Input: part model. Units: mm. Frame: model coordinates. Face numbers are marked on the shaded views. A direction names the side the tool comes from. Coordinates: 2 decimals unless noted, no trailing zeros. Loops run counter-clockwise (first coordinate to the right, second up) from the corner with the lowest first, then second, coordinate; pieces in that order, holes last. Notation, with made-up numbers: (38.25, 55.5) - (89.25, 55.5) arc R20 cw to (89.25, 72.5) - close; hole circle Ø2 at (-4.5, 1.25). An arc over 180 degrees is marked (long way). Use a Markdown table: item, result. Add a question column.
1. Draft query along X for the marked faces 3 and 4. Return one class per face: released by +X, released by -X, zero draft, split by the parting line, or undercut.
2. Section query B-B on y = 50.5. Return the cut outline in (x, z).
3. Section query C-C on y = 23. Return the cut outline in (x, z).
4. Ray query, L1, parallel to Y at x = -49, z = 1.4; L2, parallel to Y at x = -20, z = 0.55; L3, parallel to X at y = 54, z = 1.5. Return the intervals inside material, ascending. Write a range as [from, to].
5. Access query for the marked faces 1 and 2. Directions: +Z, -Z, +X, -X, +Y, -Y. A direction counts if a zero-diameter tool reaches every point of the face in a straight line with its end or side. Return the directions, or none.
6. Section query D-D on x = -4. Return the cut outline in (y, z).
7. Contact query for flat-ended pins moving along their axis: P1, Ø1, axis at x = -47.5, y = 53, coming from the +Z side; P2, Ø0.9, axis at x = -61, z = 2, coming from the -Y side; P3, Ø0.9, axis at x = -10.5, z = 1.5, coming from the -Y side; P4, Ø1.4, axis at x = -3.5, z = 1, coming from the -Y side. Output: stop coordinate, or through.
8. Section query A-A on x = -39.5. State how many separate pieces and enclosed holes the cut face has, then the cut area to 3 significant figures.
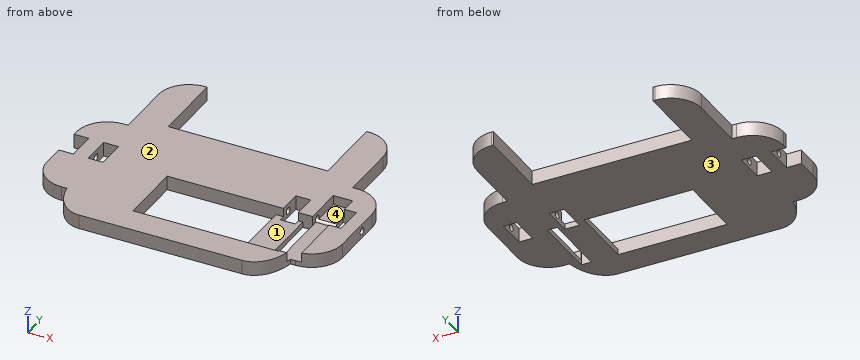
Autodesk Inventor part; units mm, degrees
ref_plane "YZ Plane" through (0, 0, 0) normal (1, 0, 0) x (0, 1, 0)
ref_plane "XZ Plane" through (0, 0, 0) normal (0, 1, 0) x (-1, 0, 0)
ref_plane "XY Plane" through (0, 0, 0) normal (0, 0, 1) x (1, 0, 0)
ref_plane "Work Plane1" through (3.6062, 5.0251, 0) normal (0, 0, 1) x (1, 0, 0)
sketch "Sketch1" plane through (3.6062, 5.0251, 0) normal (0, 0, 1) x (1, 0, 0)
  line L0 (-59.3453, 14.0249) -> (-60.5022, 14.0249)
  ellipse E0 centre (-52.8822, 15.9436) end of major axis (-52.8822, 6.6041) minor radius 6.604 (-59.3453, 14.0249) -> (-52.8822, 6.6041) ccw
  line L1 (-52.8822, 6.6041) -> (-17.8302, 6.6041)
  ellipse E1 centre (-17.8302, 15.9436) end of major axis (-17.8302, 25.2831) minor radius 6.604 (-17.8302, 6.6041) -> (-11.367, 14.0249) ccw
  line L2 (-10.2102, 14.0249) -> (-11.367, 14.0249)
  arc A0 (-10.2102, 14.0249) -> (-3.6062, 20.6289) centre (-10.2102, 20.6289) ccw
  line L3 (-3.6062, 20.6289) -> (-3.6062, 32.8209)
  arc A1 (-3.6062, 32.8209) -> (-10.2102, 39.4249) centre (-10.2102, 32.8209) ccw
  line L4 (-11.2262, 39.4249) -> (-10.2102, 39.4249)
  line L5 (-11.2262, 51.8709) -> (-11.2262, 39.4249)
  arc A2 (-11.2262, 51.8709) -> (-17.8302, 58.4749) centre (-17.8302, 51.8709) ccw
  line L6 (-17.8302, 58.4749) -> (-52.8822, 58.4749)
  arc A3 (-52.8822, 58.4749) -> (-59.4862, 51.8709) centre (-52.8822, 51.8709) ccw
  line L7 (-59.4862, 39.4249) -> (-59.4862, 51.8709)
  line L8 (-60.5022, 39.4249) -> (-59.4862, 39.4249)
  arc A4 (-60.5022, 39.4249) -> (-67.1062, 32.8209) centre (-60.5022, 32.8209) ccw
  line L9 (-67.1062, 20.6289) -> (-67.1062, 32.8209)
  arc A5 (-67.1062, 20.6289) -> (-60.5022, 14.0249) centre (-60.5022, 20.6289) ccw
  line L10 (-52.8822, 6.6041) -> (-17.8302, 6.6041)
  point P0 (-3.6062, -5.0251)
extrude "Plate1" add sketch "Sketch1" along normal blind 3.048
sketch "Sketch2" plane through (3.6062, 5.0251, 3.048) normal (0, 0, 1) x (1, 0, 0)
  line L0 (-19.2272, 69.2699) -> (-19.2272, 51.2359)
  line L1 (-42.2142, 43.5397) -> (-28.4982, 43.5397)
  line L2 (-51.4852, 51.2359) -> (-51.4852, 69.2699)
  line L3 (-19.2272, 58.5208) -> (-19.2272, 43.5397)
  line L4 (-19.2272, 43.5397) -> (-51.4852, 43.5397)
  line L5 (-51.4852, 43.5397) -> (-51.4852, 64.3147)
  line L6 (-52.4852, 58.4749) -> (-52.4852, 42.5397)
  line L7 (-52.4852, 42.5397) -> (-18.2272, 42.5397)
  line L8 (-18.2272, 42.5397) -> (-18.2272, 58.5208)
  line L9 (-52.8822, 58.4749) -> (-17.8302, 58.4749)
  point P0 (0, 0)
  point P1 (-18.2272, 58.4749)
  dimension "d2" = 1
extrude "Extrusion2" cut sketch "Sketch2" against normal through all
sketch "Sketch4" plane through (3.6062, 5.0251, 3.048) normal (0, 0, 1) x (1, 0, 0)
  line L0 (-12.8862, 21.4549) -> (-12.8862, 17.4549)
  line L1 (-9.0098, 35.2125) -> (-13.2052, 35.2125)
  line L2 (-13.2052, 35.2125) -> (-13.2052, 18.2304)
  line L3 (-13.2052, 18.2304) -> (-12.8862, 18.2304)
  line L4 (-9.0098, 16.8588) -> (-9.0098, 35.2125)
  line L5 (-9.0098, 35.2125) -> (-13.2052, 18.2304) construction
  line L6 (-13.2052, 35.2125) -> (-9.0098, 16.8588) construction
  line L7 (-12.8862, 21.4549) -> (-12.8862, 17.4549)
  line L8 (-3.6062, 30.2174) -> (-8.2582, 30.2174)
  line L9 (-12.8862, 17.9549) -> (-3.6562, 17.9549)
  line L10 (-12.8862, 21.4549) -> (-12.8862, 17.4549)
  line L11 (-13.2052, 18.2304) -> (-12.8862, 18.2304)
  line L12 (-9.0098, 16.8588) -> (-9.0098, 12.9511)
  line L13 (-9.0098, 12.9511) -> (-13.2052, 12.9511)
  line L14 (-13.2052, 12.9511) -> (-13.2052, 18.2304)
  point P0 (-3.6062, -5.0251)
  point P1 (-11.1889, 26.3919)
  point P2 (-11.1075, 26.7215)
  dimension "d18" = 4.1954
  dimension "d23" = 4.9951
  dimension "d24" = 0.3191
  dimension "d25" = 5.0038
extrude "Extrusion3" cut sketch "Sketch4" against normal blind 2
sketch "Sketch5" plane through (3.6062, 5.0251, 3.048) normal (0, 0, 1) x (1, 0, 0)
  line L0 (-52.4852, 42.5397) -> (-52.4852, 58.4749)
  line L1 (-52.8822, 58.4749) -> (-52.4852, 58.4749)
  arc A0 (-52.8822, 58.4749) -> (-59.4862, 51.8709) centre (-52.8822, 51.8709) ccw
  line L2 (-59.4862, 39.4249) -> (-59.4862, 51.8709)
  line L3 (-60.5022, 39.4249) -> (-59.4862, 39.4249)
  arc A1 (-60.5022, 39.4249) -> (-67.1062, 32.8209) centre (-60.5022, 32.8209) ccw
  line L4 (-67.1062, 20.6289) -> (-67.1062, 32.8209)
  arc A2 (-67.1062, 20.6289) -> (-60.5022, 14.0249) centre (-60.5022, 20.6289) ccw
  line L5 (-59.3453, 14.0249) -> (-60.5022, 14.0249)
  ellipse E0 centre (-52.8822, 15.9436) end of major axis (-52.8822, 6.6041) minor radius 6.604 (-59.3453, 14.0249) -> (-52.8822, 6.6041) ccw
  line L6 (-17.8302, 6.6041) -> (-52.8822, 6.6041)
  ellipse E1 centre (-17.8302, 15.9436) end of major axis (-17.8302, 25.2831) minor radius 6.604 (-17.8302, 6.6041) -> (-11.5743, 12.9511) ccw
  arc A3 (-9.0098, 14.1349) -> (-3.6062, 20.6289) centre (-10.2102, 20.6289) ccw
  line L7 (-3.6062, 32.8209) -> (-3.6062, 20.6289)
  arc A4 (-3.6062, 32.8209) -> (-10.2102, 39.4249) centre (-10.2102, 32.8209) ccw
  line L8 (-11.2262, 39.4249) -> (-10.2102, 39.4249)
  line L9 (-11.2262, 51.8709) -> (-11.2262, 39.4249)
  arc A5 (-11.2262, 51.8709) -> (-17.8302, 58.4749) centre (-17.8302, 51.8709) ccw
  line L10 (-18.2272, 58.4749) -> (-17.8302, 58.4749)
  line L11 (-18.2272, 58.4749) -> (-18.2272, 42.5397)
  line L12 (-18.2272, 42.5397) -> (-52.4852, 42.5397)
  line L13 (-13.2052, 12.9511) -> (-13.2052, 35.2125)
  line L14 (-44.45, 12.7) -> (-13.2052, 12.7)
  line L15 (-13.2052, 12.7) -> (-13.2052, 26.7215)
  line L16 (-13.2052, 26.7215) -> (-44.45, 26.7215)
  line L17 (-44.45, 26.7215) -> (-44.45, 12.7)
  line L18 (-11.5743, 12.9511) -> (-13.2052, 12.9511)
  line L19 (-13.2052, 12.9511) -> (-13.2052, 35.2125)
  line L20 (-13.2052, 35.2125) -> (-9.0098, 35.2125)
  line L21 (-9.0098, 35.2125) -> (-9.0098, 14.1349)
  point P0 (-3.6062, -5.0251)
  point P1 (-13.2052, 18.2304)
  point P2 (-41.0062, 13.5399)
  point P3 (-60.0729, 27.6299)
  dimension "d19" = 14.0215
  dimension "d20" = 31.2448
extrude "Extrusion4" cut sketch "Sketch5" against normal blind 58.7375 contours L13 L15 L14 L17 L16
sketch "Sketch6" plane through (3.6062, 5.0251, 0) normal (0, 0, -1) x (-1, 0, 0)
  line L0 (13.2052, 12.7) -> (44.45, 12.7)
  line L1 (13.2052, 26.7215) -> (44.45, 26.7215)
  line L2 (44.45, 12.7) -> (13.2052, 12.7)
  line L3 (21.1013, 12.7) -> (21.1013, 26.7215)
  line L4 (15.3165, 12.7) -> (15.3165, 26.7215)
  point P0 (3.6062, -5.0251)
extrude "Extrusion5" add sketch "Sketch6" against normal blind 1.1906
sketch "Sketch7" plane through (3.6062, 5.0251, 0) normal (0, 0, -1) x (-1, 0, 0)
  line L0 (67.1062, 25.4549) -> (67.1062, 31.8049)
  line L1 (67.1062, 31.8049) -> (63.9312, 31.8049)
  line L2 (63.9312, 31.8049) -> (63.9312, 25.4549)
  line L3 (63.9312, 25.4549) -> (67.1062, 25.4549)
  line L4 (57.5812, 31.8049) -> (57.5812, 25.4549)
  line L5 (57.5812, 25.4549) -> (60.7562, 25.4549)
  line L6 (60.7562, 25.4549) -> (60.7562, 31.8049)
  line L7 (60.7562, 31.8049) -> (57.5812, 31.8049)
  line L8 (6.4587, 31.8049) -> (6.4587, 25.4549)
  line L9 (6.4587, 25.4549) -> (9.3112, 25.4549)
  line L10 (9.3112, 25.4549) -> (9.3112, 31.8049)
  line L11 (9.3112, 31.8049) -> (6.4587, 31.8049)
  line L12 (19.4712, 25.4549) -> (19.4712, 31.8049)
  line L13 (19.4712, 31.8049) -> (16.2962, 31.8049)
  line L14 (16.2962, 31.8049) -> (16.2962, 25.4549)
  line L15 (16.2962, 25.4549) -> (19.4712, 25.4549)
  point P0 (3.6062, -5.0251)
extrude "Extrusion6" cut sketch "Sketch7" against normal blind 3.175
sketch "Sketch8" plane through (-60.325, 30.48, 0) normal (-1, 0, 0) x (0, 0, 1)
  circle A0 centre (1.4605, 3.175) radius 0.75
  point P0 (0, -30.48)
extrude "Extrusion7" cut sketch "Sketch8" against normal through all
equation "\"d5\" = Thickness"
equation "\"BendRadius\" = Thickness"
equation "\"BendReliefWidth\" = Thickness"
equation "\"BendReliefDepth\" = 0.5 * Thickness"
equation "\"CornerReliefSize\" = 4 * Thickness"
equation "\"MinimumRemnant\" = 2 * Thickness"
equation "\"TransitionRadius\" = BendRadius"
equation "\"JacobiRadiusSize\" = Thickness"
equation "\"GapSize\" = Thickness"
properties part number "_3DPrint"
Resolved:
| question | item | result |
|---|---|---|
| 1 | face 3 | zero draft |
| 1 | face 4 | undercut |
| 2 | outline | (-55.88, 0) - (-48.88, 0) - (-48.88, 3.05) - (-55.88, 3.05) - close; (-14.62, 0) - (-7.62, 0) - (-7.62, 3.05) - (-14.62, 3.05) - close |
| 3 | outline | (-62.94, 0) - (-40.84, 0) - (-40.84, 3.05) - (-62.94, 3.05) - close; (-17.5, 0) - (-11.71, 0) - (-11.71, 1.19) - (-17.5, 1.19) - close; (-9.6, 0) - (-0.56, 0) - (-0.56, 3.05) - (-5.4, 3.05) - (-5.4, 1.05) - (-9.6, 1.05) - close |
| 4 | L1 | [11.63, 32.91], [34.4, 63.5] |
| 4 | L2 | [11.63, 17.73], [31.75, 47.56] |
| 4 | L3 | [-55.88, -48.88], [-14.62, -7.62] |
| 5 | face 1 | +Z |
| 5 | face 2 | +Z, +X, -X, +Y, -Y |
| 6 | outline | (19.59, 0) - (30.48, 0) - (30.48, 3.05) - (19.59, 3.05) - close; (36.83, 0) - (43.91, 0) - (43.91, 3.05) - (36.83, 3.05) - close |
| 7 | P1 | through |
| 7 | P2 | y = 20.15 |
| 7 | P3 | y = 12.86 |
| 7 | P4 | y = 19.5 |
| 8 | separate pieces | 2 |
| 8 | enclosed holes | 1 |
| 8 | area | 65.0 mm² |
